Verification items for the finished model (mm, model axes). A direction names the side the tool comes from. Round coordinates to 2 decimals unless told otherwise and drop trailing zeros. Write each loop counter-clockwise with the first axis right and the second up, starting at its lowest first coordinate (ties: lowest second). Pieces come first, ordered by that corner, then holes. Notation, with made-up numbers: (69.25, 20.25) -> (98.25, 20.25) arc R19 ccw to (98.25, 55.25) -> close; hole circle Ø1 at (-23, 44.5). An arc over 180 degrees is marked (long way). Answer as a JSON object with one key per item and string values. Group by question number.
(1) Sectioned sample at D-D on z = -7.25. Record the cut outline in (x, y) (3 decimals), and give its area (3 significant figures).
(2) Scan lines: L1, parallel to Z at x = 1.25, y = 3; L2, parallel to Z at x = 0.75, y = -5; L3, parallel to Y at x = 0, z = -8.15 (3 decimals). Record each from-to range of solid material in increasing order. Write a range as from..to.
(3) Gauge pin test, flat ends, axial feed: pin 1 Ø6 at (y, z) = (-1.5, -4) entering from +X (3 decimals); pin 2 Ø1 at (y, z) = (-2, -3.5) entering from +X; pin 3 Ø5 at (x, y) = (0, 0.5) entering from -Z (3 decimals). Record the tip position at first contact, or that the pin passes through.
(4) Sectioned sample at A-A on y = 3.75. Record the cut outline in (x, z), and give its area (3 significant figures).
(5) Set-up check for faces 1 (the face through (0, 0, -5.715)), 2 (the face through (-0.69, -3.1, 3.92)), 3 (the face through (0, 0, 7.938)): record each of +Z, -Z, +X, -X, +Y, -Y from which the full face is reachable in a straight line by a thin tool's end or side.
(6) Draft check along Z on faces 4 (the face through (1.5, 2.8, -7.3)), 5 (the face through (-2, 3, 0.794)), 6 (the face through (-2, -3, -8.89)). Enter one of: released by +Z, released by -Z, zero draft, split by the parting line, or undercut.
```python
from build123d import *

# Parameters (mm, degrees)
SKETCH1_R           = 6.35
BOSS_EXTRUDE1_DEPTH = 0.79375
SKETCH2_R           = 3.175
BOSS_EXTRUDE2_DEPTH = 6.35
SKETCH3_R           = 6.35
BOSS_EXTRUDE3_DEPTH = 0.79375
SKETCH4_R           = 4.445
BOSS_EXTRUDE4_DEPTH = 8.89
SKETCH5_R           = 3.175
CUT_EXTRUDE1_DEPTH  = 3.175


with BuildPart() as part:
    # Sketch1 → Boss-Extrude1 (new body)
    with BuildSketch(Plane.XY):
        Circle(SKETCH1_R)
    extrude(amount=BOSS_EXTRUDE1_DEPTH)

    # Sketch2 → Boss-Extrude2 (add)
    with BuildSketch(Plane.XY.offset(0.79375)):
        Circle(SKETCH2_R)
    extrude(amount=BOSS_EXTRUDE2_DEPTH)

    # Sketch3 → Boss-Extrude3 (add)
    with BuildSketch(Plane.XY.offset(7.14375)):
        Circle(SKETCH3_R)
    extrude(amount=BOSS_EXTRUDE3_DEPTH)

    # Sketch4 → Boss-Extrude4 (add)
    with BuildSketch(Plane(origin=(0, 0, 0), x_dir=(-1, 0, 0), z_dir=(0, 0, -1))):
        Circle(SKETCH4_R)
    extrude(amount=BOSS_EXTRUDE4_DEPTH)

    # Sketch5 → Cut-Extrude1 (cut)
    with BuildSketch(Plane(origin=(0, 0, -8.89), x_dir=(-1, 0, 0), z_dir=(0, 0, -1))):
        with Locations(Location((0, 0, 0), (0, 0, 180))):
            Circle(SKETCH5_R)
    extrude(amount=-CUT_EXTRUDE1_DEPTH, mode=Mode.SUBTRACT)


solid = part.part
```
Computed values:
{
 "1": {"outline": "circle Ø8.89 at (0, 0); hole circle Ø6.35 at (0, 0)", "area": "30.4 mm2"},
 "2": {"L1": "-8.89..0.79, 7.14..7.94", "L2": "0..0.79, 7.14..7.94", "L3": "-4.445..-3.175, 3.175..4.445"},
 "3": {"pin 1": "x = 4.445", "pin 2": "x = 4.18", "pin 3": "z = -5.715"},
 "4": {"outline": "(-5.12, 0) -> (-2.39, 0) -> (-2.39, -8.89) -> (2.39, -8.89) -> (2.39, 0) -> (5.12, 0) -> (5.12, 0.79) -> (-5.12, 0.79) -> close; (-5.12, 7.14) -> (5.12, 7.14) -> (5.12, 7.94) -> (-5.12, 7.94) -> close", "area": "58.7 mm2"},
 "5": {"face 1": "-Z", "face 2": "none", "face 3": "+Z, +X, -X, +Y, -Y"},
 "6": {"face 4": "zero draft", "face 5": "undercut", "face 6": "released by -Z"}
}
